Geometry: final body of the model. Coordinates: model frame, mm. A direction names the side the tool comes from. Give positions to 0.01 mm unless a question says otherwise; leave off trailing zeros. Loops run counter-clockwise (first coordinate to the right, second up) from the corner with the lowest first, then second, coordinate; pieces in that order, holes last. Notation, with made-up numbers: M 6,-9 L 17,-9 A23 cw 17,22 Z; hole C -10.75,27.25 d10. An arc over 180 degrees is marked long. Put each result on its own line as item: value.
```python
from build123d import *

# Parameters (mm, degrees)
SKETCH1_R                 = 50.8127
BOSS_EXTRUDE1_DEPTH       = 6.35
SKETCH1_3_R               = 50.8127
SKETCH1_3_R_2             = 47.625
BOSS_EXTRUDE2_DEPTH       = 3.175
F_8_32_TAPPED_HOLE3_D     = 3.4544
F_8_32_TAPPED_HOLE3_DEPTH = 6.35
F_8_32_TAPPED_HOLE3_TIP   = 1.037806461


with BuildPart() as part:
    # Sketch1 → Boss-Extrude1 (new body)
    with BuildSketch(Plane(origin=(0, 0, 0), x_dir=(0, 0, -1), z_dir=(1, 0, 0))):
        with BuildLine():
            Line((53.975, -53.975), (53.975, 0))
            ThreePointArc((53.975, 0), (0, 53.975), (-53.975, 0))
            Line((-53.975, 0), (-53.975, -53.975))
            Line((-53.975, -53.975), (53.975, -53.975))
        make_face()
        Circle(SKETCH1_R, mode=Mode.SUBTRACT)
    extrude(amount=BOSS_EXTRUDE1_DEPTH)

    # Sketch1<3> → Boss-Extrude2 (add)
    with BuildSketch(Plane(origin=(0, 0, 0), x_dir=(0, 0, -1), z_dir=(1, 0, 0))):
        Circle(SKETCH1_3_R)
        Circle(SKETCH1_3_R_2, mode=Mode.SUBTRACT)
    extrude(amount=BOSS_EXTRUDE2_DEPTH)

    # #8-32 Tapped Hole3
    with Locations(Plane(origin=(0, -53.975, 0), x_dir=(-1, 0, 0), z_dir=(0, -1, 0))):
        with Locations((-3.175, 44.45), (-3.175, 25.4), (-3.175, -25.4), (-3.175, -44.45)):
            Hole(F_8_32_TAPPED_HOLE3_D / 2, depth=F_8_32_TAPPED_HOLE3_DEPTH)
            with Locations((0, 0, -(F_8_32_TAPPED_HOLE3_DEPTH + F_8_32_TAPPED_HOLE3_TIP / 2))):  # 118° drill point
                Cone(0, F_8_32_TAPPED_HOLE3_D / 2, F_8_32_TAPPED_HOLE3_TIP, mode=Mode.SUBTRACT)


solid = part.part
```
Item 1: Mould query, pull axis X, two halves, no side actions, for faces 4 (the cylindrical face through (2.95, -50.756, -46.163)), 5 (the flat face through (6.35, -52, 0)), 6 (the conical face through (3.04, -46.77, 44.72)), 7 (the flat face through (0, -48, 4)). Classes: pulls with the +X half, pulls with the -X half, needs draft (parallel to the pull), parting line crosses it, or undercut.
Output values:
face 4: undercut
face 5: pulls with the +X half
face 6: undercut
face 7: pulls with the -X half
Item 2: Line query: probe 1 along X at (y, z) = (-50, -25.4); probe 2 along Y at (x, z) = (4.9, 0) (3 decimals); probe 3 along Z at (x, y) = (6, -20.5) (3 decimals). Output: solid intervals per line, ascending. Write a range as [from, to].
Output values:
probe 1: [0, 1.45], [4.9, 6.35]
probe 2: [-53.975, -50.813], [50.813, 53.975]
probe 3: [-53.975, -46.494], [46.494, 53.975]
Item 3: Section B-B on y = 27.5. Output: boundary loops of the cut face in (x, z) (3 decimals).
Output values:
outline: M 0,-46.444 L 6.35,-46.444 L 6.35,-42.728 L 3.175,-42.728 L 3.175,-38.883 L 0,-38.883 Z; M 0,38.883 L 3.175,38.883 L 3.175,42.728 L 6.35,42.728 L 6.35,46.444 L 0,46.444 Z
Item 4: Set-up query: faces 1 (the cylindrical face through (1.565, -28.979, 37.794)), 2 (the cylindrical face through (2.95, -50.756, 42.737)), 3 (the flat face through (3.175, 45.4, 15.3)). Return all of +Z, -Z, +X, -X, +Y, -Y with unobstructed straight access to the full face (end or side cutting, diameter ignored); none if empty.
Output values:
face 1: +X, -X
face 2: -Y
face 3: +X
Item 5: Section A-A on z = 14. Output: boundary loops of the cut face in (x, y) (3 decimals), then the cut area to 3 significant figures.
Output values:
outline: M 0,-53.975 L 6.35,-53.975 L 6.35,-48.846 L 3.175,-48.846 L 3.175,-45.521 L 0,-45.521 Z; M 0,45.521 L 3.175,45.521 L 3.175,48.846 L 6.35,48.846 L 6.35,52.128 L 0,52.128 Z
area: 74.5 mm²
Item 6: Pin query (flat end, axial travel): pin 1 Ø1.5 at (x, y) = (4, 5) entering from -Z; pin 2 Ø1 at (x, z) = (1.5, 24) entering from +Y; pin 3 Ø2 at (x, y) = (1, 31) entering from -Z. Return the tip coordinate at first contact, or that it passes through.
Output values:
pin 1: z = -53.81
pin 2: y = 48.59
pin 3: z = -44.87
